```python
from build123d import *

# Parameters (mm, degrees)
ESQUISSE1_W             = 34.6
ESQUISSE1_H             = 64.6
BOSS_EXTRU_1_DEPTH      = 3.3
ENL_V_START             = -4.3
ESQUISSE2_W             = 8
ESQUISSE2_H             = 3.3
ENL_V_MAT_EXTRU_1_DEPTH = 5.3
ESQUISSE3_W             = 3.3
ESQUISSE3_H             = 8
ENL_V_MAT_EXTRU_2_DEPTH = 3.3


with BuildPart() as part:
    # Esquisse1 → Boss.-Extru.1 (new body)
    with BuildSketch(Plane(origin=(0, 0, 0), x_dir=(1, 0, 0), z_dir=(0, 1, 0))):
        Rectangle(ESQUISSE1_W, ESQUISSE1_H)
    extrude(amount=BOSS_EXTRU_1_DEPTH)

    # Esquisse2 → Enlèv. mat.-Extru.1 (cut)
    with BuildSketch(Plane(origin=(0, 3.3, 0), x_dir=(1, 0, 0), z_dir=(0, 1, 0)).offset(ENL_V_START)):
        with Locations((-8, 30.65)):
            Rectangle(ESQUISSE2_W, ESQUISSE2_H)
        with Locations((8, 30.65)):
            Rectangle(ESQUISSE2_W, ESQUISSE2_H)
    enl_v_mat_extru_1 = extrude(amount=ENL_V_MAT_EXTRU_1_DEPTH, mode=Mode.SUBTRACT)

    # Symétrie1: Enlèv. mat.-Extru.1 across plane
    add(enl_v_mat_extru_1.mirror(Plane.XY), mode=Mode.SUBTRACT)

    # Esquisse3 → Enlèv. mat.-Extru.2 (cut)
    with BuildSketch(Plane(origin=(0, 3.3, 0), x_dir=(1, 0, 0), z_dir=(0, 1, 0))):
        with Locations((-15.65, 0)):
            Rectangle(ESQUISSE3_W, ESQUISSE3_H)
        with Locations((-15.65, 16)):
            Rectangle(ESQUISSE3_W, ESQUISSE3_H)
        with Locations((-15.65, -16)):
            Rectangle(ESQUISSE3_W, ESQUISSE3_H)
    enl_v_mat_extru_2 = extrude(amount=-ENL_V_MAT_EXTRU_2_DEPTH, mode=Mode.SUBTRACT)

    # Symétrie2: Enlèv. mat.-Extru.2 across plane
    add(enl_v_mat_extru_2.mirror(Plane(origin=(0, 0, 0), x_dir=(0, 0, 1), z_dir=(1, 0, 0))), mode=Mode.SUBTRACT)


solid = part.part
```
Can you work these out from the model? Positions are in its coordinate system, mm. A direction names the side the tool comes from. Coordinates: 2 decimals unless noted, no trailing zeros. Order: outer loops, then holes, each group sorted by start corner. A loop starts at its lowest first (then second) coordinate and runs counter-clockwise, first axis right, second up. Notation, with made-up numbers: (23.5, -2) - (53.5, -2) arc R17 ccw to (53.5, 22) - close; hole circle Ø7 at (71, 57). An arc over 180 degrees is marked (long way). Answer in a Markdown table with one row per item.
1. Suppose I cut it at B-B (x = 5.5). Please give me the cut outline in (y, z).
Reply:
| item | result |
|---|---|
| outline | (0, -29) - (3.3, -29) - (3.3, 29) - (0, 29) - close |
2. If I drill on line 1 along Z through (x, y) = (15, 1.05); line 2 along X through (y, z) = (0.8, 19.5); line 3 along Z through (x, y) = (-6, 2.25), over which ranges is the centre line in solid material (lowest first)?
Reply:
| item | result |
|---|---|
| line 1 | z = -32.3 to -20, -12 to -4, 4 to 12, 20 to 32.3 |
| line 2 | x = -14 to 14 |
| line 3 | z = -29 to 29 |
3. For pin 1 (1.6 mm diameter, centred on x = -7, y = 1.5, fed in from +Z); pin 2 (1 mm diameter, centred on y = 1, z = 0.5, fed in from +X); pin 3 (6 mm diameter, centred on x = -13, z = 24.5, fed in from -Y); pin 4 (1 mm diameter, centred on y = 1, z = 14, fed in from -X), each with a flat end and sliding along its axis, tell me the tip position at first contact or that it passes through.
Reply:
| item | result |
|---|---|
| pin 1 | stops at z = 29 |
| pin 2 | stops at x = 14 |
| pin 3 | stops at y = 0 |
| pin 4 | stops at x = -14 |
4. If we mould it in two halves opening along X, with no side actions, what happens to faces 4 (the flat face through (-8, 2, 29)), 5 (the flat face through (0, 3.3, 0)), 6 (the flat face through (-17.3, 2, -26)), 7 (the flat face through (-8, 2, -29))? For each: pulls with the +X half, pulls with the -X half, needs draft (parallel to the pull), parting line crosses it, or undercut.
Reply:
| item | result |
|---|---|
| face 4 | undercut |
| face 5 | needs draft |
| face 6 | pulls with the -X half |
| face 7 | undercut |
5. Suppose I cut it at A-A (z = -2). Please give me the cut outline in (x, y), and give its area (3 significant figures).
Reply:
| item | result |
|---|---|
| outline | (-14, 0) - (14, 0) - (14, 3.3) - (-14, 3.3) - close |
| area | 92.4 mm^2 |
6. For faces 1 (the flat face through (4, 2, 31)), 2 (the flat face through (16, 2, -12)), 3 (the flat face through (-16, 2, 20)), which set-ups out of +Z, -Z, +X, -X, +Y, -Y let a thin tool reach every point of the face, with its end or its side?
Reply:
| item | result |
|---|---|
| face 1 | +Z, +Y, -Y |
| face 2 | +X, +Y, -Y |
| face 3 | -X, +Y, -Y |
